Build history of the part. All positions in model axes, mm. A direction names the side the tool comes from. Give positions to 0.01 mm unless a question says otherwise; leave off trailing zeros. Order: outer loops, then holes, each group sorted by start corner. A loop starts at its lowest first (then second) coordinate and runs counter-clockwise, first axis right, second up. Notation, with made-up numbers: M -2.5,79 L 11.5,79 A24 ccw 11.5,90 Z; hole C 25.5,-18 d6. An arc over 180 degrees is marked long. Answer as CSV lines item,"result".
from build123d import *

# Parameters (mm, degrees)
SKICA2_W                = 17
SKICA2_H                = 10
P_IDAT_VYSUNUT_M1_DEPTH = 5
SKICA3_W                = 17
SKICA3_H                = 0.8
P_IDAT_VYSUNUT_M2_DEPTH = 5


with BuildPart() as part:
    # Skica1 → Rotovat1 (revolve)
    with BuildSketch(Plane.XY):
        Polygon((0, 0), (0, 5), (11.5, 5), (11.5, 6.5), (23, 6.5), (23, 5), (45.5, 5), (66.5, 0.875), (66.5, 0), align=None)
    revolve(axis=Axis((0, 0, 0), (1, 0, 0)))

    # Skica2 → Přidat vysunutím1 (add)
    with BuildSketch(Plane(origin=(0, 0, 0), x_dir=(1, 0, 0), z_dir=(0, 1, 0))):
        with Locations((37, 0)):
            Rectangle(SKICA2_W, SKICA2_H)
    extrude(amount=P_IDAT_VYSUNUT_M1_DEPTH)

    # Skica3 → Přidat vysunutím2 (add)
    with BuildSketch(Plane(origin=(0, 5, 0), x_dir=(1, 0, 0), z_dir=(0, 1, 0))):
        with Locations((37, -4.6)):
            Rectangle(SKICA3_W, SKICA3_H)
        with Locations((37, 4.6)):
            Rectangle(SKICA3_W, SKICA3_H)
    extrude(amount=P_IDAT_VYSUNUT_M2_DEPTH)

    # Skica4 → Odebrat rotací1 (revolve, cut)
    with BuildSketch(Plane.XY):
        Polygon((0, 0), (0, 3.5), (45.5, 3.5), (66.5, 0.675), (66.5, 0), align=None)
    revolve(axis=Axis((0, 0, 0), (1, 0, 0)), mode=Mode.SUBTRACT)


solid = part.part
Item 1: Pull direction X, two halves, no side cores. Call faces 1 (the flat face through (28.5, 5.3, -4.5)), 2 (the flat face through (37, 5, 0)), 3 (the flat face through (11.5, -2, -5)): released by +X, released by -X, zero draft, split by the parting line, or undercut.
Geometry says:
face 1,"undercut"
face 2,"zero draft"
face 3,"released by -X"
Item 2: 3-axis set-ups, long thin cutter, end or side, ignore diameter. For faces 4 (the cylindrical face through (5.83, -1.08, -4.88)), 5 (the flat face through (37, 7, -4.2)), 6 (the flat face through (23, 2, -5)), 7 (the flat face through (37, 5, 5)), 8 (the flat face through (45.5, 5.3, 4.4)): which of +Z, -Z, +X, -X, +Y, -Y reach the whole face in a straight line?
Geometry says:
face 4,"-X"
face 5,"+X, -X, +Y"
face 6,"none"
face 7,"+Z, +X, +Y, -Y"
face 8,"+Z, +X, +Y"
Item 3: Band-saw the part on B-B (x = 7.5). Give the cut face in (y, z), and give its area (3 significant figures).
Geometry says:
outline,"C 0,0 d10; hole C 0,0 d7"
area,"40.1 mm2"
Item 4: Band-saw the part on A-A (x = 41). Give the cut face in (y, z), and give its area (3 significant figures).
Geometry says:
outline,"M 0,-5 L 10,-5 L 10,-4.2 L 5,-4.2 L 5,4.2 L 10,4.2 L 10,5 L 0,5 A5 ccw Z; hole C 0,0 d7"
area,"58.8 mm2"
Item 5: Probe line 1 along Z through (x, y) = (31, 0); line 2 along Z through (x, y) = (44.5, 6.5); line 3 along X through (y, z) = (4.5, -2.5). List the from-to ranges inside material, lowest first. Write a range as from..to.
Geometry says:
line 1,"z = -5..-3.5, 3.5..5"
line 2,"z = -5..-4.2, 4.2..5"
line 3,"x = 11.5..23, 28.5..45.5"
Item 6: Drop flat-ended pins along their axis: pin 1 (4 mm diameter, centred on y = 1.5, z = 0, fed in from +X); pin 2 (6 mm diameter, centred on x = 34, z = 0.5, fed in from +Y); pin 3 (1.5 mm diameter, centred on y = 5, z = -4.5, fed in from +X); pin 4 (5 mm diameter, centred on x = 20, y = 3.5, fed in from -Z). Give the stop position or say it passes through.
Geometry says:
pin 1,"stops at x = 66.5"
pin 2,"stops at y = 5"
pin 3,"stops at x = 45.5"
pin 4,"stops at z = -6.42"
